The listing builds one solid part. Answer for the finished solid, in the listing's coordinates (mm). A direction names the side the tool comes from. Give positions to 0.01 mm unless a question says otherwise; leave off trailing zeros. Loops run counter-clockwise (first coordinate to the right, second up) from the corner with the lowest first, then second, coordinate; pieces in that order, holes last. Notation, with made-up numbers: (84.5, 69) - (118.5, 69) arc R13 cw to (118.5, 82) - close; hole circle Ø8 at (7, 8). An arc over 180 degrees is marked (long way). Answer in a Markdown table with one row per item. Add a question column.
```python
from build123d import *

# Parameters (mm, degrees)
SKETCH7_R           = 1
BOSS_EXTRUDE1_DEPTH = 19
SKETCH8_R           = 6
BOSS_EXTRUDE2_DEPTH = 2
SKETCH9_R           = 2
BOSS_EXTRUDE3_DEPTH = 5


with BuildPart() as part:
    # Sketch7 → Boss-Extrude1 (new body)
    with BuildSketch(Plane(origin=(0, 24, 0), x_dir=(1, 0, 0), z_dir=(0, 1, 0))):
        with Locations(Location((0, 0, 0), (0, 0, 270))):
            Circle(SKETCH7_R)
    extrude(amount=BOSS_EXTRUDE1_DEPTH)

    # Sketch8 → Boss-Extrude2 (add)
    with BuildSketch(Plane(origin=(0, 43, 0), x_dir=(1, 0, 0), z_dir=(0, 1, 0))):
        with Locations(Location((0, 0, 0), (0, 0, 270))):
            Circle(SKETCH8_R)
    extrude(amount=BOSS_EXTRUDE2_DEPTH)

    # Sketch9 → Boss-Extrude3 (add)
    with BuildSketch(Plane(origin=(0, 45, 0), x_dir=(1, 0, 0), z_dir=(0, 1, 0))):
        with Locations(Location((0, 0, 0), (0, 0, 270))):
            Circle(SKETCH9_R)
    extrude(amount=BOSS_EXTRUDE3_DEPTH)

    # Sketch6 → Revolve1 (revolve)
    with BuildSketch(Plane(origin=(0, 53, 0), x_dir=(1, 0, 0), z_dir=(0, 1, 0))):
        with BuildLine():
            Line((-4, 0), (4, 0))
            ThreePointArc((4, 0), (0, 4), (-4, 0))
        make_face()
    revolve(axis=Axis((-4, 53, 0), (1, 0, 0)))


solid = part.part
```
(1) A tool of negligible diameter and unlimited length cuts with its end or side. For faces 4 (the face through (-1, 33, 0)), 5 (the face through (-2, 47, 0)), from which of +Z, -Z, +X, -X, +Y, -Y can it reach the whole face along a straight path? Write none if from no direction.
(2) A cutting plane is placed at D-D on x = 5. Determine the outline of the cut face in (y, z).
(3) A cutting plane is placed at B-B on z = 0. Determine the outline of the cut face in (x, y), plus the area to 3 significant figures.
(4) The mould has two halves that part along Y. Classify faces 1 (the face through (0, 45, 3)), 2 (the face through (0, 24, 0)), 3 (the face through (1.802, 43.986, 5.723)): pulls with the +Y half, pulls with the -Y half, needs draft (parallel to the pull), parting line crosses it, or undercut.
(5) Find the intervals of material crossed by line 1 along Y through (x, z) = (-5, 0.25); line 2 along Y through (x, z) = (3, -0.25); line 3 along Z through (x, y) = (-0.5, 31), in increasing order. Write a range as [from, to].
(6) A cutting plane is placed at C-C on y = 46. Determine the outline of the cut face in (x, z).
(7) A cutting plane is placed at A-A on x = -3.5. Determine the outline of the cut face in (y, z), plus the area to 3 significant figures.
(8) Given pin 1 Ø4 at (x, z) = (4, -3.5) entering from -Y; pin 2 Ø2 at (y, z) = (45, -3.5) entering from +X; pin 3 Ø3 at (y, z) = (45.5, -4) entering from -X; pin 4 Ø6 at (x, z) = (2, -0.5) entering from -Y, each flat-ended and moving along its own axis, determine where each tip first touches the part or whether it passes through.
Evaluation:
| question | item | result |
|---|---|---|
| 1 | face 4 | -Y |
| 1 | face 5 | none |
| 2 | outline | (43, -3.32) - (45, -3.32) - (45, 3.32) - (43, 3.32) - close |
| 3 | outline | (-6, 43) - (-1, 43) - (-1, 24) - (1, 24) - (1, 43) - (6, 43) - (6, 45) - (2, 45) - (2, 49.54) arc R4 ccw (long way) to (-2, 49.54) - (-2, 45) - (-6, 45) - close |
| 3 | area | 129 mm² |
| 4 | face 1 | undercut |
| 4 | face 2 | pulls with the -Y half |
| 4 | face 3 | needs draft |
| 5 | line 1 | y = [43, 45] |
| 5 | line 2 | y = [43, 45], [50.37, 55.63] |
| 5 | line 3 | z = [-0.87, 0.87] |
| 6 | outline | circle Ø4 at (0, 0) |
| 7 | outline | (43, -4.87) - (45, -4.87) - (45, 4.87) - (43, 4.87) - close; circle Ø3.87 at (53, 0) |
| 7 | area | 31.3 mm² |
| 8 | pin 1 | stops at y = 43 |
| 8 | pin 2 | stops at x = 5.45 |
| 8 | pin 3 | stops at x = -5.41 |
| 8 | pin 4 | stops at y = 24 |
